Here's the drawing with two shaded views (mm, measured from the low corner). I have some questions. A direction names the side the tool comes from. Coordinates: 2 decimals unless noted, no trailing zeros. Write each loop counter-clockwise with the first axis right and the second up, starting at its lowest first coordinate (ties: lowest second). Pieces come first, ordered by that corner, then holes.
Item 1: Thinking about a two-plate mould opening in Z: for the marked faces 6, 7 and 8, which applies, +Z half, -Z half, draft (parallel to the pull), parting line (faces both ways), or undercut?
Item 2: I want a section at B-B on z = 22.5. Please give me the cut outline in (x, y), then the cut area to 3 significant figures.
Item 3: If I drill on probe 1 along X at (y, z) = (4.4, 5); probe 2 along X at (y, z) = (2.95, 15.5) (1 decimal); probe 3 along Z at (x, y) = (26, 1.15) (1 decimal), over which ranges is the centre line in solid material (lowest first)?
Item 4: I want a section at C-C on x = 8.5. Please give me the cut outline in (y, z).
Item 5: Which directions (+Z, -Z, +X, -X, +Y, -Y) give clear straight access to the entire face, cutting with the end or side of a thin tool? Please do the marked faces 1, 2, 3, 4 and 5.
Item 6: I want a section at D-D on y = 1.7. State how many separate pieces and enclosed holes the cut face has, then the cut area to 3 significant figures.
Item 7: I want a section at A-A on x = 17.5. Please give me the cut outline in (y, z).
Item 8: For P1, Ø2, axis at y = 4, z = 5.5, coming from the +X side, with a flat end and sliding along its axis, tell me the tip position at first contact or that it passes through.
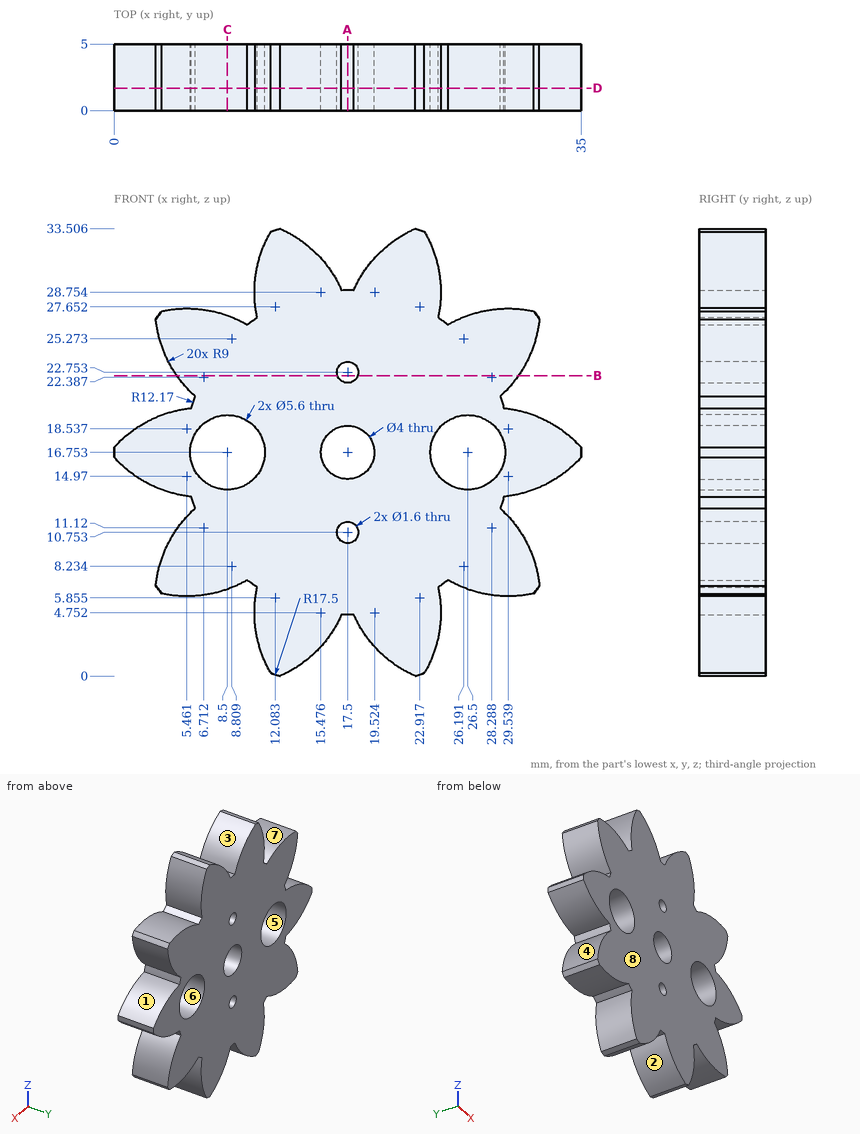
Response values:
1. face 6: undercut
1. face 7: +Z half
1. face 8: draft
2. outline: (4.7, 0) - (16.74, 0) - (16.74, 5) - (4.7, 5) - close; (18.26, 0) - (30.3, 0) - (30.3, 5) - (18.26, 5) - close
2. area: 120 mm2
3. probe 1: x = 10.53 to 24.47
3. probe 2: x = 0.9 to 6, 11 to 15.9, 19.1 to 24, 29 to 34.1
3. probe 3: z = 6.7 to 14, 19.5 to 26.8
4. outline: (0, 6.5) - (5, 6.5) - (5, 13.95) - (0, 13.95) - close; (0, 19.55) - (5, 19.55) - (5, 27.01) - (0, 27.01) - close
5. face 1: +X, +Y, -Y
5. face 2: -Z, +Y, -Y
5. face 3: +Z, +Y, -Y
5. face 4: -X, +Y, -Y
5. face 5: +Y, -Y
6. separate pieces: 1
6. enclosed holes: 5
6. area: 645 mm2
7. outline: (0, 4.58) - (5, 4.58) - (5, 9.95) - (0, 9.95) - close; (0, 11.55) - (5, 11.55) - (5, 14.75) - (0, 14.75) - close; (0, 18.75) - (5, 18.75) - (5, 21.95) - (0, 21.95) - close; (0, 23.55) - (5, 23.55) - (5, 28.92) - (0, 28.92) - close
8. P1: stops at x = 31.68
